Check sheet for the modelled part. Datum: model origin and axes. Units: mm. Face numbers are marked on the shaded views. A direction names the side the tool comes from. Coordinates: 2 decimals unless noted, no trailing zeros. Loops run counter-clockwise (first coordinate to the right, second up) from the corner with the lowest first, then second, coordinate; pieces in that order, holes last. Notation, with made-up numbers: M -21,35.5 L 18,35.5 A19 cw 18,66.5 Z; hole C -36.5,-7.5 d1. An arc over 180 degrees is marked long. Write each question's results on one line, items separated by ' | '. Start each with the question number.
from build123d import *

# Parameters (mm, degrees)
BOSS_EXTRUDE1_DEPTH = 8
SKETCH2_W           = 32
SKETCH2_H           = 29.68
SKETCH2_R           = 2
BOSS_EXTRUDE2_DEPTH = 8


with BuildPart() as part:
    # Sketch1 → Boss-Extrude1 (new body)
    with BuildSketch(Plane(origin=(0, 0, 0), x_dir=(1, 0, 0), z_dir=(0, 1, 0))):
        with BuildLine():
            Line((0, 14.84), (200, 14.84))
            ThreePointArc((200, 14.84), (214.84, 0), (200, -14.84))
            Line((200, -14.84), (0, -14.84))
            Line((0, -14.84), (0, 14.84))
        make_face()
    extrude(amount=BOSS_EXTRUDE1_DEPTH)

    # Sketch2 → Boss-Extrude2 (add)
    with BuildSketch(Plane(origin=(0, 0, 0), x_dir=(1, 0, 0), z_dir=(0, 1, 0))):
        with Locations((-2, 0)):
            Rectangle(SKETCH2_W, SKETCH2_H)
        with Locations(Location((-11, 0, 0), (0, 0, 270))):
            Circle(SKETCH2_R, mode=Mode.SUBTRACT)
    extrude(amount=-BOSS_EXTRUDE2_DEPTH)


solid = part.part
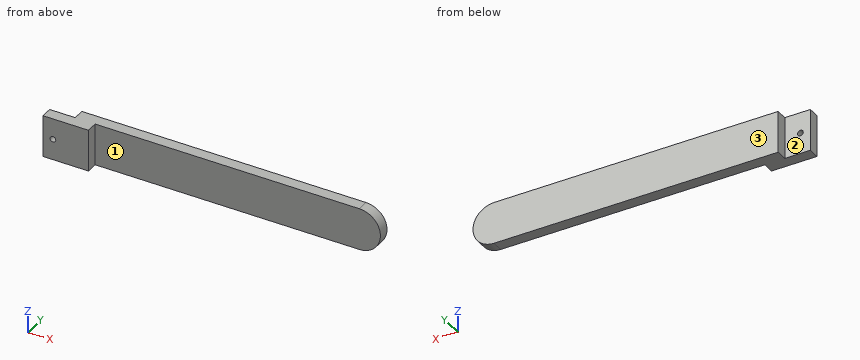
Item 1: Section check B-B (x = -11). Record the cut outline in (y, z), plus the area to 3 significant figures.
Item 2: Section check D-D (y = 5.75). Record the cut outline in (x, z).
Item 3: Section check A-A (z = 0). Record the cut outline in (x, y), plus the area to 3 significant figures.
Item 4: Section check C-C (z = 9.75). Record the cut outline in (x, y), plus the area to 3 significant figures.
Item 5: Depth check by flat-ended pin: P1, Ø5, axis at x = 116, z = 3, coming from the -Y side; P2, Ø9, axis at x = -8, z = -6, coming from the +Y side; P3, Ø1.5, axis at y = 2, z = 5.5, coming from the +X side. Enter the tip coordinate at first touch or a pass-through.
Item 6: Tool access check on the marked faces 1, 2 and 3. Record the directions out of +Z, -Z, +X, -X, +Y, -Y that give a thin tool (end or side, any length) a straight path to the whole face; none if there is none.
Item 7: Thickness scan on line 1 (X direction, y = -5.75, z = 0); line 2 (Y direction, x = 110, z = -3.5); line 3 (X direction, y = -4, z = 2.25). Record the ranges inside material, lowest first.
Computed values:
1) outline: M -8,-14.84 L 0,-14.84 L 0,-2 L -8,-2 Z; M -8,2 L 0,2 L 0,14.84 L -8,14.84 Z | area: 205 mm²
2) outline: M 0,-14.84 L 200,-14.84 A14.84 ccw 200,14.84 L 0,14.84 Z
3) outline: M -18,-8 L -13,-8 L -13,0 L -18,0 Z; M -9,-8 L 14,-8 L 14,0 L 214.84,0 L 214.84,8 L 0,8 L 0,0 L -9,0 Z | area: 1,940 mm²
4) outline: M -18,-8 L 14,-8 L 14,0 L 211.19,0 L 211.19,8 L 0,8 L 0,0 L -18,0 Z | area: 1,950 mm²
5) P1: stops at y = 0 | P2: stops at y = 0 | P3: stops at x = 214.06
6) face 1: +Z, -Z, +X, -Y | face 2: +Z, -Z, -X, +Y | face 3: +Z, -Z, +X, -X, +Y
7) line 1: x = -18 to -13, -9 to 14 | line 2: y = 0 to 8 | line 3: x = -18 to 14
